from build123d import *

# Parameters (mm, degrees)
EXTRUDE_1_DEPTH      = 40
FILLET_1_R           = 1
FILLET_2_R           = 10
FILLET_3_R           = 15
SHELL_1_T            = -4
EXTRUDE_2_REACH      = 101.561
EXTRUDE_2_END_RADIUS = 32.5
SKETCH_3_W           = 4
SKETCH_3_H           = 32
FILLET_4_R           = 6
EXTRUDE_3_DEPTH      = 2
EXTRUDE_3_DEPTH_BACK = 2
EXTRUDE_3_START      = -20


with BuildPart() as part:
    # 草图1 → 凸台-拉伸1 (new body)
    with BuildSketch(Plane.XY):
        with BuildLine():
            Line((-32.5, -106.75), (32.5, -106.75))
            Line((32.5, -106.75), (32.5, -96.75))
            Line((32.5, -96.75), (20, -96.75))
            Line((20, -96.75), (20, -20.303940504))
            ThreePointArc((20, -20.303940504), (0, -28.5), (-20, -20.303940504))
            Line((-20, -20.303940504), (-20, -96.75))
            Line((-20, -96.75), (-32.5, -96.75))
            Line((-32.5, -96.75), (-32.5, -106.75))
        make_face()
    extrude(amount=EXTRUDE_1_DEPTH)

    # 圆角1
    fillet_1_edges = [part.edges().sort_by_distance(p)[0] for p in [
        (-20, -20.303940504, 20),
        (20, -20.303940504, 20),
    ]]
    fillet(fillet_1_edges, radius=FILLET_1_R)

    # 圆角2
    fillet_2_edges = [part.edges().sort_by_distance(p)[0] for p in [
        (32.5, -96.75, 20),
        (-32.5, -96.75, 20),
    ]]
    fillet(fillet_2_edges, radius=FILLET_2_R - 0.0001)  # a hair under: the kernel refuses the full size

    # 圆角3
    fillet_3_edges = [part.edges().sort_by_distance(p)[0] for p in [
        (20, -96.75, 20),
        (-20, -96.75, 20),
    ]]
    fillet(fillet_3_edges, radius=FILLET_3_R)

    # 抽壳1
    shell_1_openings = [part.faces().sort_by_distance(p)[0] for p in [
        (0, -106.75, 20),
    ]]
    offset(amount=SHELL_1_T, openings=shell_1_openings)

    # 凸台-拉伸2: up to this cylinder (the profile starts outside it)
    extrude_2_end = Plane(origin=(0, 0, 20), z_dir=(0, 0, -1)) * Cylinder(EXTRUDE_2_END_RADIUS, 269.122, mode=Mode.PRIVATE)
    # 草图3 → 凸台-拉伸2 (add, up to the surface)
    with BuildSketch(Plane.XZ.offset(106.75), mode=Mode.PRIVATE) as extrude_2_sk1:
        with Locations((0, 20)):
            Rectangle(SKETCH_3_W, SKETCH_3_H)
    extrude_2_tool1 = extrude(extrude_2_sk1.sketch, amount=-EXTRUDE_2_REACH, mode=Mode.PRIVATE) - extrude_2_end
    add(extrude_2_tool1.solids().sort_by_distance((0, -106.75, 20))[0])

    # 圆角4
    fillet_4_edges = [part.edges().sort_by_distance(p)[0] for p in [
        (16, -28.28869032, 20),
        (-16, -28.28869032, 20),
        (-2, -32.438403167, 20),
        (2, -32.438403167, 20),
    ]]
    fillet(fillet_4_edges, radius=FILLET_4_R)

    # 草图5 → 凸台-拉伸3 (add, two sides: drawn at the far end of the back side and taken through both)
    with BuildSketch(Plane.XY.offset(40).offset(EXTRUDE_3_START - EXTRUDE_3_DEPTH_BACK)):
        with BuildLine():
            Line((-32.5, -106.75), (32.5, -106.75))
            ThreePointArc((32.5, -106.75), (31.160254038, -101.75), (27.5, -98.089745962))
            ThreePointArc((27.5, -98.089745962), (22.009618943, -92.599364905), (20, -85.099364905))
            Line((20, -85.099364905), (20, -22.566568193))
            ThreePointArc((20, -22.566568193), (19.421860287, -21.659907342), (18.355932203, -21.801599779))
            ThreePointArc((18.355932203, -21.801599779), (0, -28.5), (-18.355932203, -21.801599779))
            ThreePointArc((-18.355932203, -21.801599779), (-19.421860287, -21.659907342), (-20, -22.566568193))
            Line((-20, -22.566568193), (-20, -85.099364905))
            ThreePointArc((-20, -85.099364905), (-22.009618943, -92.599364905), (-27.5, -98.089745962))
            ThreePointArc((-27.5, -98.089745962), (-31.160254038, -101.75), (-32.5, -106.75))
        make_face()
    extrude(amount=EXTRUDE_3_DEPTH + EXTRUDE_3_DEPTH_BACK)


solid = part.part
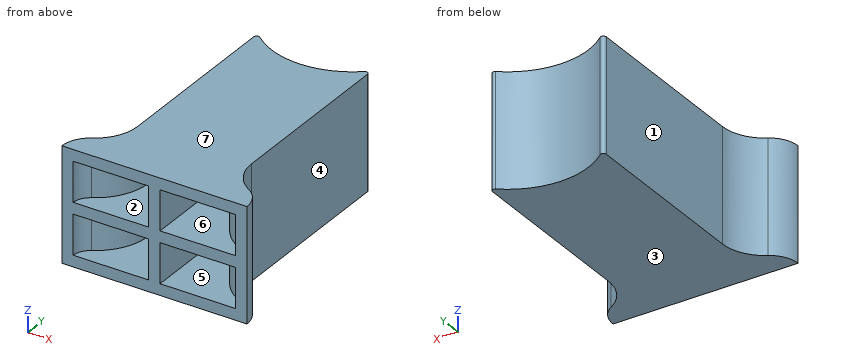
Part model, mm, in its own coordinate system. Face numbers are marked on the shaded views. A direction names the side the tool comes from. Round coordinates to 2 decimals unless told otherwise and drop trailing zeros. Loops run counter-clockwise (first coordinate to the right, second up) from the corner with the lowest first, then second, coordinate; pieces in that order, holes last. Notation, with made-up numbers: (23.5, -23) - (71.5, -23) arc R11 ccw to (71.5, -2) - close; hole circle Ø7 at (47, 76). An arc over 180 degrees is marked (long way). Answer as a JSON object with one key per item and string values.
Item 1: Pin check, flat tips, straight feed: pin 1 (4 mm diameter, centred on y = -65, z = 26.5, fed in from -X); pin 2 (3 mm diameter, centred on y = -43, z = 8, fed in from +X); pin 3 (1 mm diameter, centred on x = -25, z = 15, fed in from -Y); pin 4 (6 mm diameter, centred on x = -24, y = -51, fed in from +Z). Stop position of each tip, or through.
Output:
{"pin 1": "x = -20", "pin 2": "x = 20", "pin 3": "y = -101.55", "pin 4": "through"}
Item 2: Tool access for the marked faces 1, 2 and 3: list every direction of +Z, -Z, +X, -X, +Y, -Y with a clear straight run to the whole face (end or side of a thin tool).
Output:
{"face 1": "+Z, -Z, -X, +Y", "face 2": "-Y", "face 3": "-Z, +X, -X, +Y, -Y"}
Item 3: Band-saw the part on B-B on y = -27.5. List the corners of the cut face in (x, z), plus the area to 3 significant figures.
Output:
{"outline": "(-20, 0) - (-7.48, 0) - (-7.48, 40) - (-20, 40) - close; (7.48, 0) - (20, 0) - (20, 40) - (7.48, 40) - close", "area": "1,000 mm2"}
Item 4: Band-saw the part on D-D on x = 15. List the corners of the cut face in (y, z), plus the area to 3 significant figures.
Output:
{"outline": "(-106.75, 0) - (-24.23, 0) - (-24.23, 40) - (-106.75, 40) - (-106.75, 36) - (-33.86, 36) - (-33.86, 22) - (-106.75, 22) - (-106.75, 18) - (-33.86, 18) - (-33.86, 4) - (-106.75, 4) - close", "area": "1,260 mm2"}
Item 5: Band-saw the part on C-C on x = -14.5. List the corners of the cut face in (y, z).
Output:
{"outline": "(-106.75, 0) - (-24.54, 0) - (-24.54, 40) - (-106.75, 40) - (-106.75, 36) - (-33.21, 36) - (-33.21, 22) - (-106.75, 22) - (-106.75, 18) - (-33.21, 18) - (-33.21, 4) - (-106.75, 4) - close"}
Item 6: Pull direction X, two halves, no side cores. Call the marked faces 4, 5, 6 and 7: pulls with the +X half, pulls with the -X half, needs draft (parallel to the pull), parting line crosses it, or undercut.
Output:
{"face 4": "pulls with the +X half", "face 5": "undercut", "face 6": "undercut", "face 7": "needs draft"}
Item 7: Band-saw the part on A-A on y = -80. List the corners of the cut face in (x, z), plus the area to 3 significant figures.
Output:
{"outline": "(-20, 0) - (20, 0) - (20, 40) - (-20, 40) - close; hole (-16, 4) - (-2, 4) - (-2, 18) - (-16, 18) - close; hole (-16, 22) - (-2, 22) - (-2, 36) - (-16, 36) - close; hole (2, 4) - (16, 4) - (16, 18) - (2, 18) - close; hole (2, 22) - (16, 22) - (16, 36) - (2, 36) - close", "area": "816 mm2"}
Item 8: Wall check: L1, parallel to X at y = -39.5, z = 10.5; L2, parallel to Z at x = -9.5, y = -34; L3, parallel to X at y = -102, z = 32. Give the ranges that are in metal, low to high.
Output:
{"L1": "-20 to -16, -2 to 2, 16 to 20", "L2": "0 to 4, 18 to 22, 36 to 40", "L3": "-31.3 to -26.17, -2 to 2, 26.17 to 31.3"}
